Read the model definition and answer for the solid it produces. Units are mm, in the model's axes. Face numbers are marked on the shaded views. A direction names the side the tool comes from. Round coordinates to 2 decimals unless told otherwise and drop trailing zeros. Order: outer loops, then holes, each group sorted by start corner. A loop starts at its lowest first (then second) coordinate and runs counter-clockwise, first axis right, second up. Notation, with made-up numbers: (-32, 37.5) -> (-12, 37.5) arc R17 ccw to (-12, 52.5) -> close; hole circle Ø6 at (-4, 65.5). An arc over 180 degrees is marked (long way). One line per item, written item: value. Start each with the question number.
1. Section A-A (x = 0) is taken. Give the vertices of the cut face in (y, z).
2. Section D-D (z = 4.25) is taken. Give the vertices of the cut face in (x, y).
3. Consider line 1 (Z direction, x = -3.75, y = -3.5); line 2 (Z direction, x = 0, y = -6); line 3 (X direction, y = -3, z = 7). Determine where each line is inside the solid, lowest interval first.
4. Flat-ended cylindrical pins translate along their axes: pin 1 Ø5 at (x, y) = (0, 0) entering from +Z; pin 2 Ø1.5 at (x, z) = (5, 8) entering from -Y; pin 3 Ø4 at (x, z) = (-3, 7) entering from +Y. Find the tip coordinate at first contact, or state that the pin passes through.
5. Section C-C (z = 8.25) is taken. Give the vertices of the cut face in (x, y).
6. Section B-B (y = 0) is taken. Give the vertices of the cut face in (x, z), then the cut area to 4 significant figures.
7. The mould has two halves that part along Y. Classify the marked faces 1, 2, 3 and 4: released by +Y, released by -Y, zero draft, split by the parting line, or undercut.
8. For the marked faces 5, 6 and 7, determine the directions among +Z, -Z, +X, -X, +Y, -Y from which every point of the face is accessible in a straight line to the end or side of a thin tool.
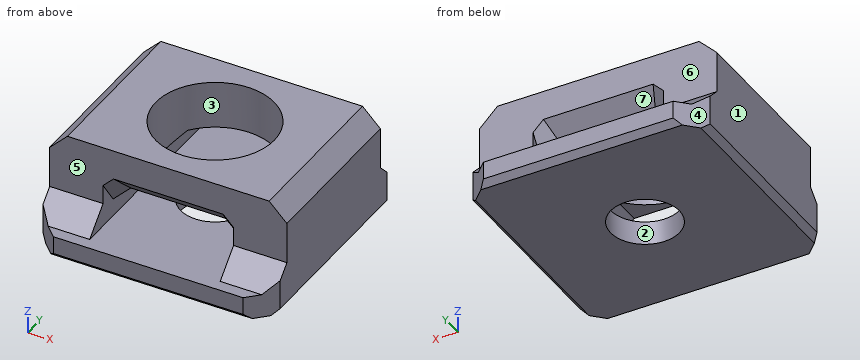
Autodesk Inventor part; units mm, degrees
ref_plane "YZ Plane" through (0, 0, 0) normal (1, 0, 0) x (0, 1, 0)
ref_plane "XZ Plane" through (0, 0, 0) normal (0, 1, 0) x (-1, 0, 0)
ref_plane "XY Plane" through (0, 0, 0) normal (0, 0, 1) x (1, 0, 0)
sketch "Sketch1" plane through (0, 0, 0) normal (0, 0, 1) x (1, 0, 0)
  line L0 (-10, -10) -> (10, -10)
  line L1 (10, -10) -> (10, 10)
  line L2 (10, 10) -> (-10, 10)
  line L3 (-10, 10) -> (-10, -10)
  line L4 (-10, -10) -> (10, 10) construction
  line L5 (10, -10) -> (-10, 10) construction
  circle A0 centre (0, 0) radius 2.9
  dimension "d0" = 20
  dimension "d1" = 20
  dimension "d2" = 5.8
extrude "Extrusion1" add sketch "Sketch1" along normal blind 2
chamfer "Chamfer1" distance 0.5 angle 45 4 edges at (10, 0, 0) (0, 10, 0) (-10, 0, 0) (0, -10, 0)
sketch "Sketch2" plane through (0, 0, 2) normal (0, 0, 1) x (1, 0, 0)
  line L0 (10, 10) -> (10, -10)
  line L1 (-10, -7) -> (10, -7)
  line L2 (10, -7) -> (10, 7)
  line L3 (10, 7) -> (-10, 7)
  line L4 (-10, 7) -> (-10, -7)
  line L5 (-10, -7) -> (10, 7) construction
  line L6 (10, -7) -> (-10, 7) construction
  point P0 (0, 0)
  dimension "d8" = 14
extrude "Extrusion2" add sketch "Sketch2" along normal blind 7
sketch "Sketch5" plane through (-10, -7, 2) normal (0, -1, 0) x (1, 0, 0)
  line L0 (20, 0) -> (0, 0)
  line L1 (4.5, 0) -> (15.5, 0)
  line L2 (15.5, 0) -> (15.5, 3)
  line L3 (15.5, 3) -> (4.5, 3)
  line L4 (4.5, 3) -> (4.5, 0)
  line L5 (0, 0) -> (0, 7)
  line L6 (20, 0) -> (20, 7)
  point P0 (10, -2)
  dimension "d18" = 3
  dimension "d19" = 4.5
  dimension "d20" = 4.5
extrude "Extrusion4" cut sketch "Sketch5" against normal through all
sketch "Sketch6" plane through (0, 0, 9) normal (0, 0, 1) x (1, 0, 0)
  circle A0 centre (0, 0) radius 2.9 construction
  circle A1 centre (0, 0) radius 5
  dimension "d23" = 10
extrude "Extrusion5" cut sketch "Sketch6" against normal up to surface (7 mm away)
chamfer "Chamfer4" distance 1.5 angle 45 2 edges at (-5.5, 0, 5) (5.5, 0, 5)
chamfer "Chamfer5" distance 1.5 angle 45 6 edges at (0, -7, 5) (0, 7, 5) (-4.75, -7, 4.25) (4.75, -7, 4.25) (4.75, 7, 4.25) (-4.75, 7, 4.25)
chamfer "Chamfer6" distance 1.5 angle 45 2 edges at (-10, 0, 9) (10, 0, 9)
chamfer "Chamfer7" distance 2 angle 45 8 edges at (10, 10, 1.25) (-10, 10, 1.25) (-10, -10, 1.25) (10, -10, 1.25) (7.75, -7, 2) (-7.75, -7, 2) (-7.75, 7, 2) (7.75, 7, 2)
equation "\"d20\" = d19"
properties part number "_3DPrint"
Answer:
1. outline: (-10, 0.5) -> (-9.5, 0) -> (-2.9, 0) -> (-2.9, 2) -> (-10, 2) -> close; (-7, 6.5) -> (-5.5, 5) -> (-5, 5) -> (-5, 9) -> (-7, 9) -> close; (2.9, 0) -> (9.5, 0) -> (10, 0.5) -> (10, 2) -> (2.9, 2) -> close; (5, 5) -> (5.5, 5) -> (7, 6.5) -> (7, 9) -> (5, 9) -> close
2. outline: (-10, -7) -> (-5.5, -7) -> (-5.5, -6.03) -> (-4.75, -5.5) -> (-4.75, -1.56) arc R5 cw to (-4.75, 1.56) -> (-4.75, 5.5) -> (-5.5, 6.03) -> (-5.5, 7) -> (-10, 7) -> close; (4.75, -5.5) -> (5.5, -6.03) -> (5.5, -7) -> (10, -7) -> (10, 7) -> (5.5, 7) -> (5.5, 6.03) -> (4.75, 5.5) -> (4.75, 1.56) arc R5 cw to (4.75, -1.56) -> close
3. line 1: 0 to 2, 5 to 9
3. line 2: 0 to 2, 5.5 to 9
3. line 3: -10 to -4, 4 to 10
4. pin 1: through
4. pin 2: y = -7
4. pin 3: y = 7
5. outline: (-9.25, -7) -> (9.25, -7) -> (9.25, 7) -> (-9.25, 7) -> close; hole circle Ø10 at (0, 0)
6. outline: (-10, 0.5) -> (-9.5, 0) -> (-2.9, 0) -> (-2.9, 2) -> (-5.5, 2) -> (-5.5, 3.5) -> (-5, 4) -> (-5, 9) -> (-8.5, 9) -> (-10, 7.5) -> close; (2.9, 0) -> (9.5, 0) -> (10, 0.5) -> (10, 7.5) -> (8.5, 9) -> (5, 9) -> (5, 4) -> (5.5, 3.5) -> (5.5, 2) -> (2.9, 2) -> close
6. area: 94.15 mm^2
7. face 1: zero draft
7. face 2: undercut
7. face 3: undercut
7. face 4: released by +Y
8. face 5: +Z, +X, -X, -Y
8. face 6: +Z, +X, -X, +Y
8. face 7: +Y
